Source: CAD feature listing. Evaluate the final solid. Frame: model axes, mm. A direction names the side the tool comes from. Give positions to 0.01 mm unless a question says otherwise; leave off trailing zeros. Order: outer loops, then holes, each group sorted by start corner. A loop starts at its lowest first (then second) coordinate and runs counter-clockwise, first axis right, second up. Notation, with made-up numbers: (26.5, 72.25) - (44.5, 72.25) arc R28 ccw to (44.5, 91.25) - close; hole circle Ø4 at (35.5, 74). An arc over 180 degrees is marked (long way). One line per item, written item: value. Start each with the question number.
from build123d import *

# Parameters (mm, degrees)
SKETCH1_W                = 14
SKETCH1_H                = 18
BOSS_EXTRUDE1_DEPTH      = 1
BOSS_EXTRUDE2_DEPTH      = 2
BOSS_EXTRUDE2_DEPTH_BACK = 5
SKETCH2_W                = 5.78
SKETCH2_H                = 2.56


with BuildPart() as part:
    # Sketch1 → Boss-Extrude1 (new body)
    with BuildSketch(Plane(origin=(0, 0, 0), x_dir=(1, 0, 0), z_dir=(0, 1, 0))):
        with Locations((7, -9)):
            Rectangle(SKETCH1_W, SKETCH1_H)
    extrude(amount=BOSS_EXTRUDE1_DEPTH)

    # Sketch2 → Boss-Extrude2 (add, two sides: drawn at the far end of the back side and taken through both)
    with BuildSketch(Plane.XY.offset(18).offset(-BOSS_EXTRUDE2_DEPTH_BACK)):
        with BuildLine():
            Line((4.11, 3.56), (4.11, 1))
            ThreePointArc((4.11, 1), (2.83, 2.28), (4.11, 3.56))
        make_face()
        with Locations((7, 2.28)):
            Rectangle(SKETCH2_W, SKETCH2_H)
        with BuildLine():
            ThreePointArc((9.89, 3.56), (11.17, 2.28), (9.89, 1))
            Line((9.89, 1), (9.89, 3.56))
        make_face()
    extrude(amount=BOSS_EXTRUDE2_DEPTH + BOSS_EXTRUDE2_DEPTH_BACK)


solid = part.part
1. Set-up query: faces 1 (the flat face through (7, 1, 19)), 2 (the flat face through (7, 2, 13)), 3 (the flat face through (14, 0.5, 9.1)). Return all of +Z, -Z, +X, -X, +Y, -Y with unobstructed straight access to the full face (end or side cutting, diameter ignored); none if empty.
2. Ray query, L1, parallel to Z at x = 10.25, y = 0.9; L2, parallel to Y at x = 11.5, z = 4; L3, parallel to Z at x = 10.5, y = 1.6. Return the intervals inside material, ascending.
3. Draft query along Y for faces 4 (the cylindrical face through (11.17, 2.31, 16.45)), 5 (the flat face through (7, 3.56, 16)), 6 (the flat face through (6.9, 0.5, 18)). Return one class per face: pulls with the +Y half, pulls with the -Y half, needs draft (parallel to the pull), parting line crosses it, or undercut.
4. Contact query for flat-ended pins moving along their axis: pin 1 Ø1 at (x, z) = (6, 19.5) entering from -Y; pin 2 Ø0.8 at (x, y) = (5.5, 0.5) entering from +Z; pin 3 Ø0.8 at (x, y) = (8.5, 1.5) entering from -Z. Output: stop coordinate, or through.
5. Section A-A on x = 5.5. Return the cut outline in (y, z).
6. Section B-B on z = 3.5. Return the cut outline in (x, y).
7. Section C-C on y = 2.28. Return the cut outline in (x, z).
Data:
1. face 1: +Z, +X, -X, -Y
1. face 2: -Z, +X, -X, +Y
1. face 3: +Z, -Z, +X, +Y, -Y
2. L1: z = 0 to 18
2. L2: y = 0 to 1
2. L3: z = 13 to 20
3. face 4: undercut
3. face 5: pulls with the +Y half
3. face 6: needs draft
4. pin 1: stops at y = 1
4. pin 2: stops at z = 18
4. pin 3: stops at z = 13
5. outline: (0, 0) - (1, 0) - (1, 13) - (3.56, 13) - (3.56, 20) - (1, 20) - (1, 18) - (0, 18) - close
6. outline: (0, 0) - (14, 0) - (14, 1) - (0, 1) - close
7. outline: (2.83, 13) - (11.17, 13) - (11.17, 20) - (2.83, 20) - close
